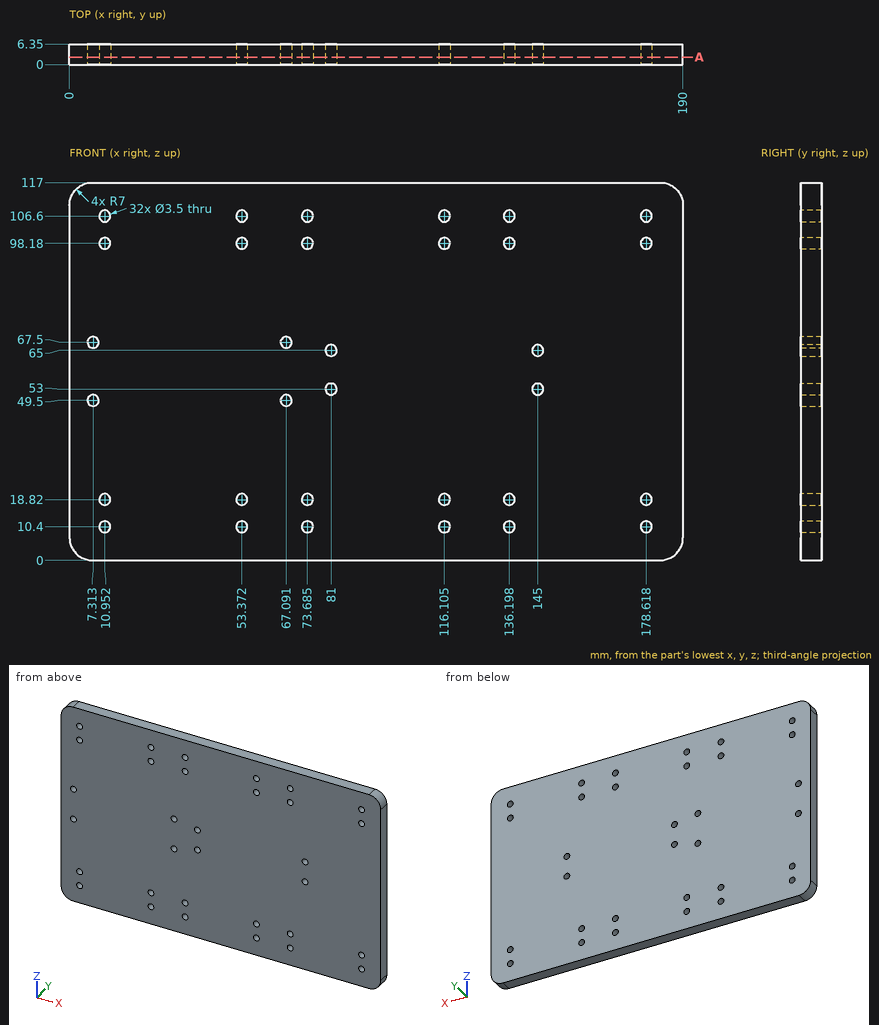
Print and shaded views of the part. All mm, measured from the part's lowest x, y and z. Round coordinates to 2 decimals unless told otherwise and drop trailing zeros. Use CSV: the item, a comma, the result in double quotes. Start each with the question number.
Item 1: Drill centre lines: L1, parallel to X at y = 4.75, z = 67.5; L2, parallel to Z at x = 81, y = 4.5; L3, parallel to Z at x = 137, y = 2.75 (1 decimal). Where is each one in solid material? Low to high. Write a range as [from, to].
Item 2: Pin check, flat tip, straight feed: P1, Ø4.5, axis at x = 81, z = 53, coming from the -Y side. Stop position of the tip, or through.
Item 3: Band-saw the part on A-A (y = 2.25). State how many separate pieces and enclosed holes the cut face has, and give its area (3 significant figures).
Checked values:
1,L1,"x = [0, 5.56], [9.06, 65.34], [68.84, 190]"
1,L2,"z = [0, 51.25], [54.75, 63.25], [66.75, 117]"
1,L3,"z = [0, 8.8], [12, 17.3], [20.4, 96.6], [99.7, 105], [108.2, 117]"
2,P1,"stops at y = 0"
3,separate pieces,"1"
3,enclosed holes,"32"
3,area,"21,900 mm²"
